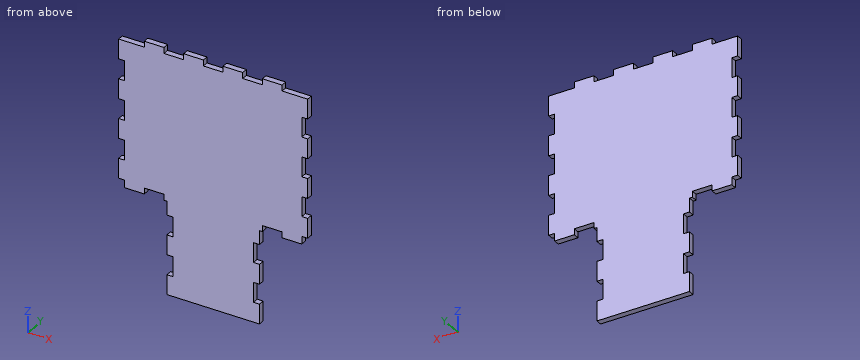
from build123d import *

# Parameters (mm, degrees)
BOSS_EXTRUDE1_DEPTH     = 3
SKETCH3_W               = 10
SKETCH3_H               = 3
BOSS_EXTRUDE2_DEPTH     = 3
LPATTERN1_COUNT         = 3
LPATTERN1_PITCH         = 20
SKETCH4_W               = 10
SKETCH4_H               = 3
BOSS_EXTRUDE3_DEPTH     = 3
LPATTERN2_COUNT         = 2
LPATTERN2_PITCH         = 20
SKETCH5_W               = 10
SKETCH5_H               = 3
BOSS_EXTRUDE4_DEPTH     = 3
LPATTERN3_COUNT         = 4
LPATTERN3_PITCH         = 20
SKETCH6_W               = 10
SKETCH6_H               = 3
BOSS_EXTRUDE5_DEPTH     = 3
LPATTERN4_COUNT         = 2
LPATTERN4_PITCH         = 20
MIRROR3_COPY_1_SKETCH_W = 10
MIRROR3_COPY_1_SKETCH_H = 3
MIRROR3_COPY_1_DEPTH    = 3
MIRROR3_COPY_2_SKETCH_W = 10
MIRROR3_COPY_2_SKETCH_H = 3
MIRROR3_COPY_2_DEPTH    = 3
MIRROR3_COPY_3_SKETCH_W = 10
MIRROR3_COPY_3_SKETCH_H = 3
MIRROR3_COPY_3_DEPTH    = 3
MIRROR3_COPY_4_SKETCH_W = 10
MIRROR3_COPY_4_SKETCH_H = 3
MIRROR3_COPY_4_DEPTH    = 3
MIRROR3_COPY_5_SKETCH_W = 10
MIRROR3_COPY_5_SKETCH_H = 3
MIRROR3_COPY_5_DEPTH    = 3
MIRROR3_COPY_6_SKETCH_W = 10
MIRROR3_COPY_6_SKETCH_H = 3
MIRROR3_COPY_6_DEPTH    = 3
MIRROR3_COPY_7_SKETCH_W = 10
MIRROR3_COPY_7_SKETCH_H = 3
MIRROR3_COPY_7_DEPTH    = 3


with BuildPart() as part:
    # Sketch1 → Boss-Extrude1 (new body)
    with BuildSketch(Plane(origin=(0, 0, 0), x_dir=(1, 0, 0), z_dir=(0, 1, 0))):
        Polygon((20.5, 60.804597701), (-20.5, 60.804597701), (-20.5, 10.804597701), (-45, 10.804597701), (-45, -60.045977011), (45, -60.045977011), (45, 10.804597701), (20.5, 10.804597701), align=None)
    extrude(amount=BOSS_EXTRUDE1_DEPTH)

    # Sketch3 → Boss-Extrude2 (add)
    with BuildSketch(Plane.ZY.offset(20.5)):
        with Locations((-55.804597701, 1.5)):
            Rectangle(SKETCH3_W, SKETCH3_H)
    boss_extrude2 = extrude(amount=BOSS_EXTRUDE2_DEPTH)

    # LPattern1: Boss-Extrude2 ×3
    with Locations(*[(0, 0, i * LPATTERN1_PITCH) for i in range(1, LPATTERN1_COUNT)]):
        add(boss_extrude2)

    # Sketch4 → Boss-Extrude3 (add)
    with BuildSketch(Plane(origin=(0, 0, -10.804597701), x_dir=(-1, 0, 0), z_dir=(0, 0, -1))):
        with Locations((-40, 1.5)):
            Rectangle(SKETCH4_W, SKETCH4_H)
    boss_extrude3 = extrude(amount=BOSS_EXTRUDE3_DEPTH)

    # LPattern2: Boss-Extrude3 ×2
    with Locations(*[(-i * LPATTERN2_PITCH, 0, 0) for i in range(1, LPATTERN2_COUNT)]):
        add(boss_extrude3)

    # Sketch5 → Boss-Extrude4 (add)
    with BuildSketch(Plane(origin=(45, 0, 0), x_dir=(0, 0, -1), z_dir=(1, 0, 0))):
        with Locations((-55.045977011, 1.5)):
            Rectangle(SKETCH5_W, SKETCH5_H)
    boss_extrude4 = extrude(amount=BOSS_EXTRUDE4_DEPTH)

    # LPattern3: Boss-Extrude4 ×4
    with Locations(*[(0, 0, -i * LPATTERN3_PITCH) for i in range(1, LPATTERN3_COUNT)]):
        add(boss_extrude4)

    # Sketch6 → Boss-Extrude5 (add)
    with BuildSketch(Plane.XY.offset(60.045977011)):
        with Locations((10, 1.5)):
            Rectangle(SKETCH6_W, SKETCH6_H)
    boss_extrude5 = extrude(amount=BOSS_EXTRUDE5_DEPTH)

    # LPattern4: Boss-Extrude5 ×2
    with Locations(*[(i * LPATTERN4_PITCH, 0, 0) for i in range(1, LPATTERN4_COUNT)]):
        add(boss_extrude5)

    # Mirror3: Boss-Extrude2, Boss-Extrude3, Boss-Extrude4, Boss-Extrude5 across plane
    add(boss_extrude2.mirror(Plane.ZY))
    add(boss_extrude3.mirror(Plane.ZY))
    add(boss_extrude4.mirror(Plane.ZY))
    add(boss_extrude5.mirror(Plane.ZY))

    # Mirror3 copy 1 sketch → Mirror3 copy 1 (add)
    with BuildSketch(Plane(origin=(20, 0, -10.804597701), x_dir=(1, 0, 0), z_dir=(0, 0, -1))):
        with Locations((-40, -1.5)):
            Rectangle(MIRROR3_COPY_1_SKETCH_W, MIRROR3_COPY_1_SKETCH_H)
    extrude(amount=MIRROR3_COPY_1_DEPTH)

    # Mirror3 copy 2 sketch → Mirror3 copy 2 (add)
    with BuildSketch(Plane(origin=(-20, 0, 60.045977011), x_dir=(-1, 0, 0), z_dir=(0, 0, 1))):
        with Locations((10, -1.5)):
            Rectangle(MIRROR3_COPY_2_SKETCH_W, MIRROR3_COPY_2_SKETCH_H)
    extrude(amount=MIRROR3_COPY_2_DEPTH)

    # Mirror3 copy 3 sketch → Mirror3 copy 3 (add)
    with BuildSketch(Plane(origin=(-45, 0, -20), x_dir=(0, 0, -1), z_dir=(-1, 0, 0))):
        with Locations((-55.045977011, -1.5)):
            Rectangle(MIRROR3_COPY_3_SKETCH_W, MIRROR3_COPY_3_SKETCH_H)
    extrude(amount=MIRROR3_COPY_3_DEPTH)

    # Mirror3 copy 4 sketch → Mirror3 copy 4 (add)
    with BuildSketch(Plane(origin=(-45, 0, -40), x_dir=(0, 0, -1), z_dir=(-1, 0, 0))):
        with Locations((-55.045977011, -1.5)):
            Rectangle(MIRROR3_COPY_4_SKETCH_W, MIRROR3_COPY_4_SKETCH_H)
    extrude(amount=MIRROR3_COPY_4_DEPTH)

    # Mirror3 copy 5 sketch → Mirror3 copy 5 (add)
    with BuildSketch(Plane(origin=(-45, 0, -60), x_dir=(0, 0, -1), z_dir=(-1, 0, 0))):
        with Locations((-55.045977011, -1.5)):
            Rectangle(MIRROR3_COPY_5_SKETCH_W, MIRROR3_COPY_5_SKETCH_H)
    extrude(amount=MIRROR3_COPY_5_DEPTH)

    # Mirror3 copy 6 sketch → Mirror3 copy 6 (add)
    with BuildSketch(Plane(origin=(20.5, 0, 20), x_dir=(0, 0, 1), z_dir=(1, 0, 0))):
        with Locations((-55.804597701, -1.5)):
            Rectangle(MIRROR3_COPY_6_SKETCH_W, MIRROR3_COPY_6_SKETCH_H)
    extrude(amount=MIRROR3_COPY_6_DEPTH)

    # Mirror3 copy 7 sketch → Mirror3 copy 7 (add)
    with BuildSketch(Plane(origin=(20.5, 0, 40), x_dir=(0, 0, 1), z_dir=(1, 0, 0))):
        with Locations((-55.804597701, -1.5)):
            Rectangle(MIRROR3_COPY_7_SKETCH_W, MIRROR3_COPY_7_SKETCH_H)
    extrude(amount=MIRROR3_COPY_7_DEPTH)


solid = part.part
Check sheet for the modelled part. Datum: model origin and axes. Units: mm. Give positions to 0.01 mm unless a question says otherwise; leave off trailing zeros. Write each loop counter-clockwise with the first axis right and the second up, starting at its lowest first coordinate (ties: lowest second). Pieces come first, ordered by that corner, then holes. Notation, with made-up numbers: (73, -10) -> (86, -10) arc R22 cw to (86, -2) -> close; hole circle Ø4 at (-12.75, 10). An arc over 180 degrees is marked (long way). Use one line per item in the form item = value. Start each with the question number.
1. Thickness scan on line 1 along X through (y, z) = (1.8, -16.5); line 2 along Z through (x, y) = (-41, 0.9); line 3 along Z through (x, y) = (26, 0.6). Record the ranges inside material, lowest first. Write a range as from..to.
2. Section check B-B (z = 47). Record the cut outline in (x, y).
3. Go/stop test with flat-tipped pins: P1, Ø0.9, axis at x = -38.5, y = 2, coming from the -Z side; P2, Ø0.9, axis at x = 22.5, y = 2, coming from the +Z side; P3, Ø0.9, axis at y = 2, z = 44.5, coming from the -X side. Record where each tip stops, or that it passes through.
4. Section check A-A (x = -2). Record the cut outline in (y, z), and give its area (3 significant figures).
Conclusion:
q1.line_1 = -23.5..23.5
q1.line_2 = -13.8..60.05
q1.line_3 = -10.8..63.05
q2.outline = (-45, 0) -> (45, 0) -> (45, 3) -> (-45, 3) -> close
q3.P1 = -13.8
q3.P2 = 60.05
q3.P3 = -45
q4.outline = (0, -60.8) -> (3, -60.8) -> (3, 60.05) -> (0, 60.05) -> close
q4.area = 363 mm²
